Autodesk Fusion 360 part; units mm, degrees
sketch "Sketch1" plane through (0, 0, 0) normal (0, 0, 1) x (1, 0, 0)
  line L0 (7.8365, 56.717) -> (95.1165, 56.717)
  line L1 (95.1165, 56.717) -> (99.132, 0.6987)
  line L2 (99.132, 0.6987) -> (2.632, 0.6987)
  line L3 (2.632, 0.6987) -> (7.8365, 56.717)
  dimension "d1" = 87.28
  dimension "d2" = 96.5
  dimension "d3" = 95.308
  dimension "d4" = 94.1
extrude "Extrude1" add sketch "Sketch1" along normal blind 3
sketch "Sketch2" plane through (0, 56.717, 0) normal (0, 1, 0) x (-1, 0, 0)
  line L0 (-95.1165, 0) -> (-7.8365, 0)
  line L1 (-7.8365, 0) -> (-7.8365, 3)
  line L2 (-7.8365, 3) -> (-95.1165, 3)
  line L3 (-95.1165, 3) -> (-95.1165, 0)
  line L4 (-92.1095, 3) -> (-92.1095, 16)
  line L5 (-92.1095, 16) -> (-76.1095, 16)
  line L6 (-76.1095, 16) -> (-76.1095, 3)
  line L7 (-69.6275, 3) -> (-69.6275, 16)
  line L8 (-69.6275, 16) -> (-53.6275, 16)
  line L9 (-53.6275, 16) -> (-53.6275, 3)
  line L10 (-47.1465, 3) -> (-47.1465, 16)
  line L11 (-47.1465, 16) -> (-31.1465, 16)
  line L12 (-31.1465, 16) -> (-31.1465, 3)
  line L13 (-27.0655, 3) -> (-27.0655, 16)
  line L14 (-27.0655, 16) -> (-11.0655, 16)
  line L15 (-11.0655, 16) -> (-11.0655, 3)
  line L16 (-74.6095, 17.5) -> (-74.6095, 3)
  line L17 (-71.1275, 3) -> (-71.1275, 17.5)
  line L18 (-48.6465, 3) -> (-48.6465, 17.5)
  line L19 (-48.6465, 17.5) -> (-29.6465, 17.5)
  line L20 (-29.6465, 17.5) -> (-29.6465, 3)
  line L21 (-28.5655, 3) -> (-28.5655, 17.5)
  line L22 (-28.5655, 17.5) -> (-9.5655, 17.5)
  line L23 (-9.5655, 17.5) -> (-9.5655, 3)
  line L24 (-74.6095, 17.5) -> (-93.6095, 17.5)
  line L25 (-93.6095, 17.5) -> (-93.6095, 3)
  line L26 (-71.1275, 17.5) -> (-52.1275, 17.5)
  line L27 (-52.1275, 17.5) -> (-52.1275, 3)
  dimension "d7" = 3.007
  dimension "d11" = 16
  dimension "d12" = 6.482
  dimension "d13" = 16
  dimension "d14" = 6.481
  dimension "d15" = 16
  dimension "d16" = 4.081
  dimension "d17" = 16
  dimension "d18" = 13
  dimension "d19" = 13
  dimension "d20" = 13
  dimension "d21" = 13
  dimension "d23" = 1.5
  dimension "d24" = 1.5
  dimension "d25" = 1.5
  dimension "d26" = 1.5
  dimension "d28" = 1.5
  dimension "d29" = 1.5
  dimension "d30" = 1.5
  dimension "d31" = 1.5
  dimension "d32" = 1.5
  dimension "d33" = 1.5
  dimension "d34" = 1.5
  dimension "d35" = 1.5
extrude "Extrude2" add sketch "Sketch2" against normal blind 40 from surface at -5 contours L2 L4 L5 L6 L16 L24 L25 | L2 L13 L14 L15 L21 L22 L23 | L2 L7 L8 L9 L17 L26 L27 | L2 L10 L11 L12 L18 L19 L20
sketch "Sketch3" plane through (0, 56.717, 0) normal (0, 1, 0) x (-1, 0, 0)
  line L0 (-95.1165, 0) -> (-7.8365, 0)
  line L1 (-7.8365, 0) -> (-7.8365, 3)
  line L2 (-7.8365, 3) -> (-95.1165, 3)
  line L3 (-95.1165, 3) -> (-95.1165, 0)
  line L4 (-92.1095, 3) -> (-76.1095, 3)
  line L5 (-76.1095, 0) -> (-92.1095, 0)
  line L6 (-92.1095, 3) -> (-92.1095, 0)
  line L7 (-76.1095, 3) -> (-76.1095, 0)
  line L8 (-69.6275, 3) -> (-69.6275, 0)
  line L9 (-69.6275, 3) -> (-53.6275, 3)
  line L10 (-53.6275, 0) -> (-53.6275, 3)
  line L11 (-53.6275, 0) -> (-69.6275, 0)
  line L12 (-47.1465, 3) -> (-47.1465, 0)
  line L13 (-47.1465, 3) -> (-31.1465, 3)
  line L14 (-31.1465, 0) -> (-31.1465, 3)
  line L15 (-31.1465, 0) -> (-47.1465, 0)
  line L16 (-27.0925, 3) -> (-11.0925, 3)
  line L17 (-11.0925, 0) -> (-11.0925, 3)
  line L18 (-11.0925, 0) -> (-27.0925, 0)
  line L19 (-27.0925, 3) -> (-27.0925, 0)
  dimension "d39" = 16
  dimension "d40" = 16
  dimension "d41" = 16
  dimension "d42" = 16
  dimension "d43" = 3.007
  dimension "d44" = 6.482
  dimension "d45" = 6.481
  dimension "d46" = 4.054
extrude "Extrude3" cut sketch "Sketch3" against normal blind 51 contours L0 L2 L4 L5 L6 L7 | L0 L2 L8 L9 L10 L11 | L0 L2 L12 L13 L14 L15 | L0 L2 L16 L17 L18 L19
fillet "Fillet1" radius 2.5 1 edges at (93.6095, 31.717, 17.5)
fillet "Fillet2" radius 2.5 7 edges at (74.6095, 31.717, 17.5) (71.1275, 31.717, 17.5) (52.1275, 31.717, 17.5) (48.6465, 31.717, 17.5) (29.6465, 31.717, 17.5) (9.5655, 31.717, 17.5) (28.5655, 31.717, 17.5)
fillet "Fillet3" radius 1 1 edges at (50.882, 0.6987, 3)
fillet "Fillet4" radius 1.5 2 edges at (27.0655, 31.717, 16) (11.0655, 31.717, 16)
fillet "Fillet4" radius 1.5 6 edges at (31.1465, 31.717, 16) (53.6275, 31.717, 16) (76.1095, 31.717, 16) (47.1465, 31.717, 16) (69.6275, 31.717, 16) (92.1095, 31.717, 16)
sketch "Sketch4" plane through (0, 0, 3) normal (0, 0, 1) x (-1, 0, 0)
  line L0 (-9.5655, -11.717) -> (-9.5655, -51.717)
  line L1 (-9.5655, -51.717) -> (-11.0655, -51.717)
  line L2 (-11.0655, -51.717) -> (-11.0655, -11.717)
  line L3 (-11.0655, -11.717) -> (-9.5655, -11.717)
  line L4 (-2.7249, -1.6987) -> (-99.0603, -1.6987)
  line L5 (-99.0603, -1.6987) -> (-95.1165, -56.717)
  line L6 (-95.1165, -56.717) -> (-92.1095, -56.717)
  line L7 (-92.1095, -56.717) -> (-92.1095, -51.717)
  line L8 (-92.1095, -51.717) -> (-93.6095, -51.717)
  line L9 (-93.6095, -51.717) -> (-93.6095, -11.717)
  line L10 (-93.6095, -11.717) -> (-92.1095, -11.717)
  line L11 (-92.1095, -11.717) -> (-92.1095, -5.717)
  line L12 (-92.1095, -5.717) -> (-76.1095, -5.717)
  line L13 (-76.1095, -5.717) -> (-76.1095, -11.717)
  line L14 (-76.1095, -11.717) -> (-74.6095, -11.717)
  line L15 (-74.6095, -11.717) -> (-74.6095, -51.717)
  line L16 (-74.6095, -51.717) -> (-76.1095, -51.717)
  line L17 (-76.1095, -51.717) -> (-76.1095, -56.717)
  line L18 (-76.1095, -56.717) -> (-69.6275, -56.717)
  line L19 (-69.6275, -56.717) -> (-69.6275, -51.717)
  line L20 (-69.6275, -51.717) -> (-71.1275, -51.717)
  line L21 (-71.1275, -51.717) -> (-71.1275, -11.717)
  line L22 (-71.1275, -11.717) -> (-69.6275, -11.717)
  line L23 (-69.6275, -11.717) -> (-69.6275, -5.717)
  line L24 (-69.6275, -5.717) -> (-53.6275, -5.717)
  line L25 (-53.6275, -5.717) -> (-53.6275, -11.717)
  line L26 (-53.6275, -11.717) -> (-52.1275, -11.717)
  line L27 (-52.1275, -11.717) -> (-52.1275, -51.717)
  line L28 (-52.1275, -51.717) -> (-53.6275, -51.717)
  line L29 (-53.6275, -51.717) -> (-53.6275, -56.717)
  line L30 (-53.6275, -56.717) -> (-47.1465, -56.717)
  line L31 (-47.1465, -56.717) -> (-47.1465, -51.717)
  line L32 (-47.1465, -51.717) -> (-48.6465, -51.717)
  line L33 (-48.6465, -51.717) -> (-48.6465, -11.717)
  line L34 (-48.6465, -11.717) -> (-47.1465, -11.717)
  line L35 (-47.1465, -11.717) -> (-47.1465, -5.717)
  line L36 (-47.1465, -5.717) -> (-31.1465, -5.717)
  line L37 (-31.1465, -5.717) -> (-31.1465, -11.717)
  line L38 (-31.1465, -11.717) -> (-29.6465, -11.717)
  line L39 (-29.6465, -11.717) -> (-29.6465, -51.717)
  line L40 (-29.6465, -51.717) -> (-31.1465, -51.717)
  line L41 (-31.1465, -51.717) -> (-31.1465, -56.717)
  line L42 (-31.1465, -56.717) -> (-27.0925, -56.717)
  line L43 (-27.0925, -56.717) -> (-27.0925, -51.717)
  line L44 (-27.0925, -51.717) -> (-28.5655, -51.717)
  line L45 (-28.5655, -51.717) -> (-28.5655, -11.717)
  line L46 (-28.5655, -11.717) -> (-27.0925, -11.717)
  line L47 (-27.0925, -11.717) -> (-27.0925, -5.717)
  line L48 (-27.0925, -5.717) -> (-11.0925, -5.717)
  line L49 (-11.0925, -5.717) -> (-11.0925, -56.717)
  line L50 (-11.0925, -56.717) -> (-7.8365, -56.717)
  line L51 (-7.8365, -56.717) -> (-2.7249, -1.6987)
  circle A0 centre (-50.1165, -53.717) radius 0.6186
  circle A1 centre (-6.7249, -3.717) radius 0.5
  circle A2 centre (-95.0603, -3.717) radius 0.5
  circle A3 centre (-50.3865, -7.717) radius 0.5
  dimension "d59" = 3
  dimension "d60" = 3.511
  dimension "d61" = 1
  dimension "d63" = 2
  dimension "d64" = 4
  dimension "d65" = 1
  dimension "d66" = 4
  dimension "d67" = 2
  dimension "d68" = 1
  dimension "d69" = 3.24
  dimension "d70" = 2
hole "Hole1" at (50.1165, 53.717, 3) at (6.7249, 3.717, 3) at (50.3865, 7.717, 3) at (95.0603, 3.717, 3) direction (0, 0, -1) diameter 1 depth 1.5 tip angle 118
Geometry: final body of the model. Coordinates: model frame, mm. A direction names the side the tool comes from. Round coordinates to 2 decimals unless told otherwise and drop trailing zeros. Order: outer loops, then holes, each group sorted by start corner. A loop starts at its lowest first (then second) coordinate and runs counter-clockwise, first axis right, second up. Notation, with made-up numbers: (35, 81) -> (61, 81) arc R32 ccw to (61, 111) -> close; hole circle Ø8 at (-18.5, -21). An arc over 180 degrees is marked (long way). Use one line per item in the form item = value. Start each with the question number.
1. Cut plane B-B (z = 7.75). Count the separate pieces of the cut face and the enclosed holes in it, then the cut area to 3 significant figures.
2. Draft query along X for faces 4 (the face through (71.128, 32, 9)), 5 (the face through (62, 32, 17.5)), 6 (the face through (93.61, 32, 9)), 7 (the face through (62, 32, 16)). Return one class per face: pulls with the +X half, pulls with the -X half, needs draft (parallel to the pull), parting line crosses it, or undercut.
3. Pin query (flat end, axial travel): pin 1 Ø2.5 at (y, z) = (18.5, 2) entering from -X; pin 2 Ø4 at (y, z) = (44.5, 10.5) entering from +X; pin 3 Ø2.5 at (x, z) = (18, 1) entering from +Y; pin 4 Ø4 at (x, y) = (72.5, 40) entering from -Z. Return the tip coordinate at first contact, or that it passes through.
4. Reachability of faces 1 (the face through (27.092, 32, 2)), 2 (the face through (84.2, 11.717, 16.2)), 3 (the face through (27.9, 31.4, 16.7)) from +Z, -Z, +X, -X, +Y, -Y: full face, straight path, thin tool, end or side. Return the list, or none.
5. Line query: probe 1 along X at (y, z) = (16, 16.75); probe 2 along Z at (x, y) = (72, 45.5); probe 3 along Z at (x, y) = (45, 36.5). Output: solid intervals per line, ascending.
6. Cut plane A-A (x = 16.5). Return the cut outline in (y, z), then the cut area to 3 significant figures.
Solution:
q1.separate_pieces = 8
q1.enclosed_holes = 0
q1.area = 480 mm^2
q2.face_4 = undercut
q2.face_5 = needs draft
q2.face_6 = pulls with the +X half
q2.face_7 = undercut
q3.pin_1 = 4.17
q3.pin_2 = 93.61
q3.pin_3 = 5.72
q3.pin_4 = 0
q4.face_1 = -Z, +Y
q4.face_2 = +Z, +X, -X, -Y
q4.face_3 = +Z, +Y, -Y
q5.probe_1 = 10.28 to 27.85, 30.36 to 47.93, 52.84 to 70.41, 75.32 to 92.89
q5.probe_2 = 0 to 3
q5.probe_3 = 16 to 17.5
q6.outline = (0.7, 0) -> (5.72, 0) -> (5.72, 3) -> (1.7, 3) arc R1 ccw to (0.7, 2) -> close; (11.72, 16) -> (51.72, 16) -> (51.72, 17.5) -> (11.72, 17.5) -> close
q6.area = 74.8 mm^2
